Source: three-view drawing plus pictorial views. Frame: mm from the lowest corner of the part. Give positions to 0.01 mm unless a question says otherwise; leave off trailing zeros. Order: outer loops, then holes, each group sorted by start corner. A loop starts at its lowest first (then second) coordinate and runs counter-clockwise, first axis right, second up. Notation, with made-up numbers: (-24.75, 53.25) - (4.25, 53.25) arc R22 ccw to (4.25, 80.25) - close; hole circle Ø4 at (46.5, 17.25). An arc over 180 degrees is marked (long way). Answer in a Markdown table with one row per item. Add a question column.
1. Section query A-A on y = 13. Return loops of the section in (x, z), and give its area (3 significant figures).
2. Mould query, pull axis Z, two halves, no side actions, for the marked faces 1, 2 and 3. Classes: released by +Z, released by -Z, zero draft, split by the parting line, or undercut.
3. Section query C-C on z = 12.7. Return loops of the section in (x, y), and give its area (3 significant figures).
4. Ray query, line 1 (Y direction, x = 1.5, z = 12.7); line 2 (Z direction, x = 2.5, y = 12.75); line 3 (Y direction, x = 1.25, z = 10.75). Return the intervals inside material, ascending. Write a range as [from, to].
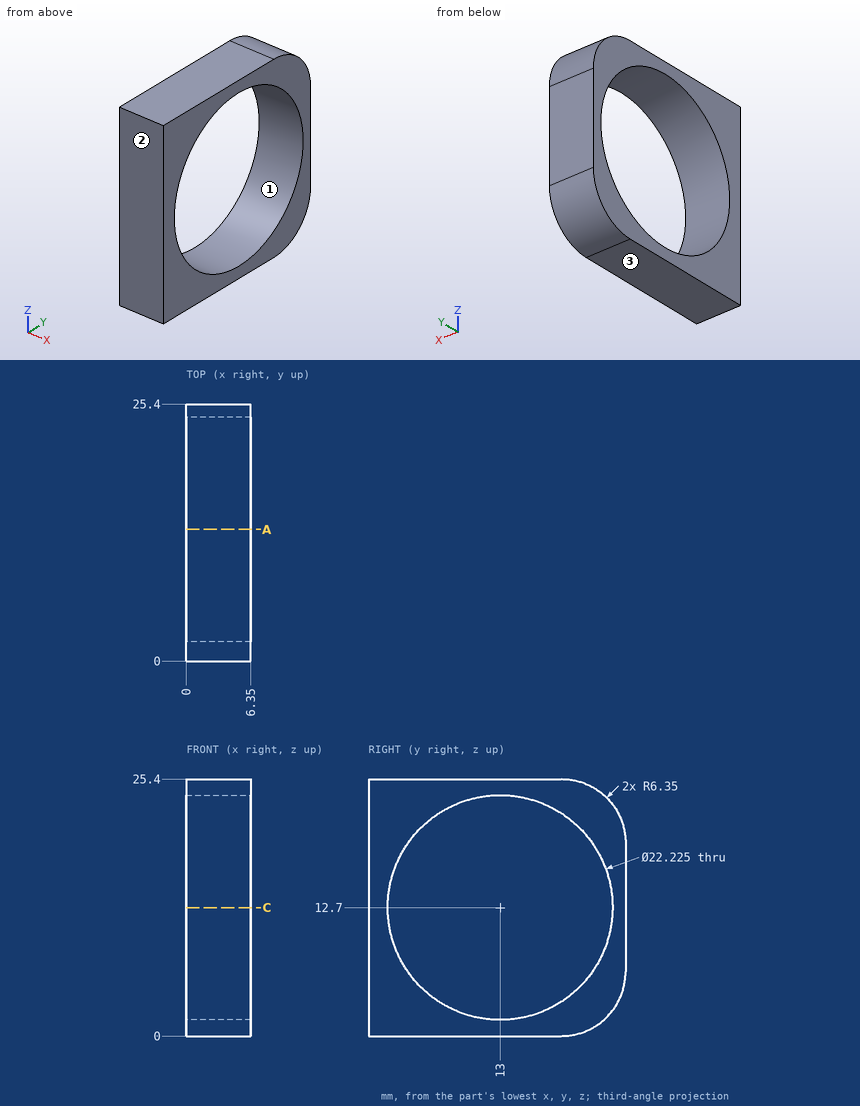
Answer:
| question | item | result |
|---|---|---|
| 1 | outline | (0, 0) - (6.35, 0) - (6.35, 1.59) - (0, 1.59) - close; (0, 23.81) - (6.35, 23.81) - (6.35, 25.4) - (0, 25.4) - close |
| 1 | area | 20.2 mm² |
| 2 | face 1 | undercut |
| 2 | face 2 | zero draft |
| 2 | face 3 | released by -Z |
| 3 | outline | (0, 0) - (6.35, 0) - (6.35, 1.89) - (0, 1.89) - close; (0, 24.11) - (6.35, 24.11) - (6.35, 25.4) - (0, 25.4) - close |
| 3 | area | 20.2 mm² |
| 4 | line 1 | y = [0, 1.89], [24.11, 25.4] |
| 4 | line 2 | z = [0, 1.59], [23.81, 25.4] |
| 4 | line 3 | y = [0, 2.06], [23.94, 25.4] |
